Print and shaded views of the part. All mm, measured from the part's lowest x, y and z. A direction names the side the tool comes from. Round coordinates to 2 decimals unless told otherwise and drop trailing zeros. Loops run counter-clockwise (first coordinate to the right, second up) from the corner with the lowest first, then second, coordinate; pieces in that order, holes last. Notation, with made-up numbers: (43, 4) -> (98, 4) arc R10 cw to (98, 12) -> close; hole circle Ø8 at (-25.75, 34). An arc over 180 degrees is marked (long way). Use a Markdown table: item, result.
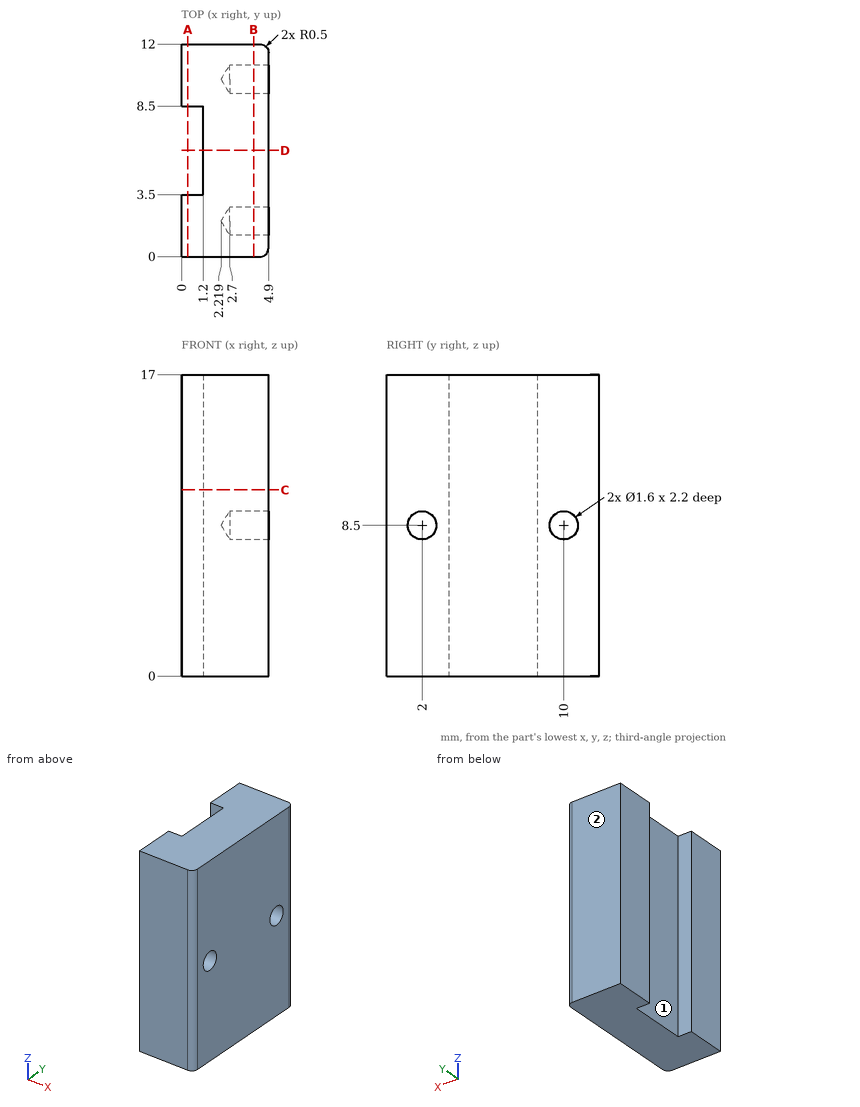
Q1. Drill centre lines: L1, parallel to Y at x = 4.45, z = 8.5; L2, parallel to Y at x = 0.95, z = 15.5; L3, parallel to Z at x = 3.55, y = 2. Where is each one in solid material? Low to high. Write a range as from..to.
Results list:
| item | result |
|---|---|
| L1 | y = 0..1.2, 2.8..9.2, 10.8..12 |
| L2 | y = 0..3.5, 8.5..12 |
| L3 | z = 0..7.7, 9.3..17 |
Q2. Band-saw the part on A-A, the plane x = 0.35. Give the cut face in (y, z), plus the area to 3 significant figures.
Results list:
| item | result |
|---|---|
| outline | (0, 0) -> (3.5, 0) -> (3.5, 17) -> (0, 17) -> close; (8.5, 0) -> (12, 0) -> (12, 17) -> (8.5, 17) -> close |
| area | 119 mm² |
Q3. Band-saw the part on B-B, the plane x = 4.05. Give the cut face in (y, z), plus the area to 3 significant figures.
Results list:
| item | result |
|---|---|
| outline | (0, 0) -> (12, 0) -> (12, 17) -> (0, 17) -> close; hole circle Ø1.6 at (2, 8.5); hole circle Ø1.6 at (10, 8.5) |
| area | 200 mm² |
Q4. Band-saw the part on D-D, the plane y = 6. Give the cut face in (x, z), plus the area to 3 significant figures.
Results list:
| item | result |
|---|---|
| outline | (1.2, 0) -> (4.9, 0) -> (4.9, 17) -> (1.2, 17) -> close |
| area | 62.9 mm² |
Q5. Tool access for the marked faces 1 and 2: list every direction of +Z, -Z, +X, -X, +Y, -Y with a clear straight run to the whole face (end or side of a thin tool).
Results list:
| item | result |
|---|---|
| face 1 | +Z, -Z, -X |
| face 2 | +Z, -Z, +X, -X, +Y |
Q6. Band-saw the part on C-C, the plane z = 10.5. Give the cut face in (x, y).
Results list:
| item | result |
|---|---|
| outline | (0, 0) -> (4.4, 0) arc R0.5 ccw to (4.9, 0.5) -> (4.9, 11.5) arc R0.5 ccw to (4.4, 12) -> (0, 12) -> (0, 8.5) -> (1.2, 8.5) -> (1.2, 3.5) -> (0, 3.5) -> close |
Q7. Flat gauge pins, fed straight in: pin 1 (2.5 mm diameter, centred on y = 7, z = 10, fed in from -X); pin 2 (1.4 mm diameter, centred on y = 2, z = 8.5, fed in from +X). Where does each tip first touch, or does it go through?
Results list:
| item | result |
|---|---|
| pin 1 | stops at x = 1.2 |
| pin 2 | stops at x = 2.64 |
